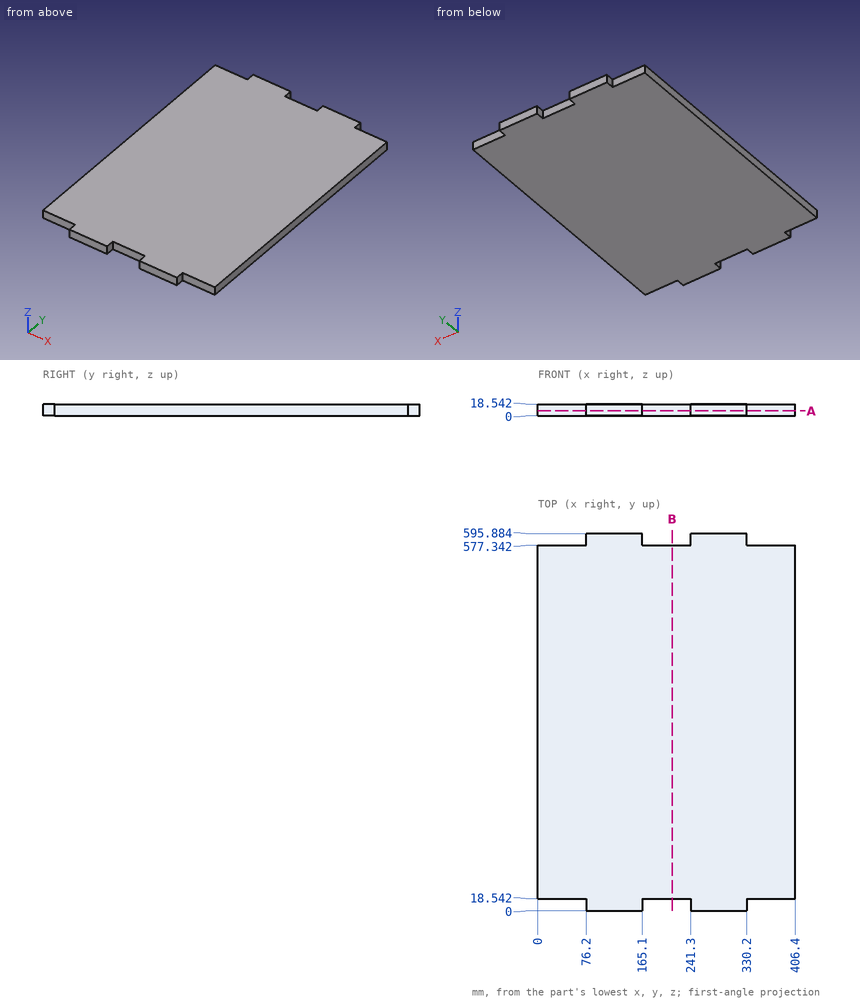
The figure shows three views and two pictorial views of one solid part (mm, origin at its lowest corner). Answer the questions. Coordinates: 2 decimals unless noted, no trailing zeros. Loops run counter-clockwise (first coordinate to the right, second up) from the corner with the lowest first, then second, coordinate; pieces in that order, holes last.
1) Flat-ended cylindrical pins translate along their axes: pin 1 Ø5.5 at (x, z) = (217, 9) entering from +Y; pin 2 Ø5.5 at (x, z) = (191.5, 12) entering from -Y; pin 3 Ø5.5 at (y, z) = (586.5, 5) entering from -X. Find the tip coordinate at first contact, or state that the pin passes through.
2) Find section A-A on z = 7.5. Write down the section's boundary in (x, y).
3) Find the intervals of material crossed by L1, parallel to Y at x = 345.5, z = 17.75, in increasing order.
4) Find section B-B on x = 212. Write down the section's boundary in (y, z), then the cut area to 3 significant figures.
Values:
1. pin 1: stops at y = 577.34
1. pin 2: stops at y = 18.54
1. pin 3: stops at x = 76.2
2. outline: (0, 18.54) - (76.2, 18.54) - (76.2, 0) - (165.1, 0) - (165.1, 18.54) - (241.3, 18.54) - (241.3, 0) - (330.2, 0) - (330.2, 18.54) - (406.4, 18.54) - (406.4, 577.34) - (330.2, 577.34) - (330.2, 595.88) - (241.3, 595.88) - (241.3, 577.34) - (165.1, 577.34) - (165.1, 595.88) - (76.2, 595.88) - (76.2, 577.34) - (0, 577.34) - close
3. L1: y = 18.54 to 577.34
4. outline: (18.54, 0) - (577.34, 0) - (577.34, 18.54) - (18.54, 18.54) - close
4. area: 10,400 mm2
